from build123d import *

# Parameters (mm, degrees)
SKETCH1_R                    = 3
BOSS_EXTRUDE1_DEPTH          = 10
SKETCH2_R                    = 6
CUT_EXTRUDE1_DEPTH           = 10
SKETCH3_R                    = 52.728139035
CUT_EXTRUDE2_DEPTH           = 10
FILLET1_R                    = 40
SKETCH4_R                    = 2.5
CUT_EXTRUDE3_DEPTH           = 10
CHAMFER1_SIZE                = 2
FILLET2_R                    = 10
LPATTERN3_COUNT              = 5
LPATTERN3_PITCH              = 40
CHAMFER1_OF_LPATTERN3_SIZE   = 2
SKETCH5_R                    = 2.5
CUT_EXTRUDE4_DEPTH           = 10
CHAMFER2_SIZE                = 2
CIRPATTERN2_COUNT            = 45
CHAMFER2_OF_CIRPATTERN2_SIZE = 2
FILLET4_R                    = 82


with BuildPart() as part:
    # Sketch1 → Boss-Extrude1 (new body)
    with BuildSketch(Plane.XY):
        with BuildLine():
            Line((134, -12.3683), (134, -2.7366))
            Line((134, -2.7366), (-66.856482862, -2.7366))
            ThreePointArc((-66.856482862, -2.7366), (-79.305955572, -8.361988007), (-74.83591229, -21.271406043))
            Line((-74.83591229, -21.271406043), (104.205340418, -118.521488224))
            ThreePointArc((104.205340418, -118.521488224), (120.331391511, -85.784656527), (130.366665775, -50.69843496))
            ThreePointArc((130.366665775, -50.69843496), (131.475070851, -44.365109618), (132.383339124, -38))
            ThreePointArc((132.383339124, -38), (133.595433619, -25.209616495), (134, -12.3683))
        make_face()
        with Locations((60, -38)):
            Circle(SKETCH1_R, mode=Mode.SUBTRACT)
        with Locations((-70, -12.3683)):
            Circle(SKETCH1_R, mode=Mode.SUBTRACT)
    extrude(amount=BOSS_EXTRUDE1_DEPTH)

    # Sketch2 → Cut-Extrude1 (cut)
    with BuildSketch(Plane.XY.offset(10)):
        with Locations((60, -38)):
            Circle(SKETCH2_R)
        with Locations((-70, -12.3683)):
            Circle(SKETCH2_R)
    extrude(amount=-CUT_EXTRUDE1_DEPTH, mode=Mode.SUBTRACT)

    # Sketch3 → Cut-Extrude2 (cut)
    with BuildSketch(Plane.XY.offset(10)):
        with Locations((-31.102013179, -89.20992017)):
            Circle(SKETCH3_R)
    extrude(amount=-CUT_EXTRUDE2_DEPTH, mode=Mode.SUBTRACT)

    # Fillet1
    fillet1_edges = [part.edges().sort_by_distance(p)[0] for p in [
        (18.78007916, -72.120932196, 5),
        (-43.920680471, -38.063674805, 5),
    ]]
    fillet(fillet1_edges, radius=FILLET1_R)

    # Sketch4 → Cut-Extrude3 (cut)
    with BuildSketch(Plane.XY.offset(10)):
        with Locations((122, -7.7366)):
            Circle(SKETCH4_R)
    cut_extrude3 = extrude(amount=-CUT_EXTRUDE3_DEPTH, mode=Mode.SUBTRACT)

    # Chamfer1
    chamfer1_edges = [part.edges().sort_by_distance(p)[0] for p in [
        (119.5, -7.7366, 10),
    ]]
    chamfer(chamfer1_edges, length=CHAMFER1_SIZE)

    # Fillet2
    fillet2_edges = [part.edges().sort_by_distance(p)[0] for p in [
        (134, -2.7366, 5),
    ]]
    fillet(fillet2_edges, radius=FILLET2_R)

    # LPattern3: Cut-Extrude3 ×5
    with Locations(*[(-i * LPATTERN3_PITCH, 0, 0) for i in range(1, LPATTERN3_COUNT)]):
        add(cut_extrude3, mode=Mode.SUBTRACT)

    # Chamfer1 of LPattern3
    chamfer1_of_lpattern3_edges = [part.edges().sort_by_distance(p)[0] for p in [
        (79.5, -7.7366, 10),
        (39.5, -7.7366, 10),
        (-0.5, -7.7366, 10),
        (-40.5, -7.7366, 10),
    ]]
    chamfer(chamfer1_of_lpattern3_edges, length=CHAMFER1_OF_LPATTERN3_SIZE)

    # Sketch5 → Cut-Extrude4 (cut)
    with BuildSketch(Plane.XY.offset(10)):
        with Locations((128.565543545, -25.510785173)):
            Circle(SKETCH5_R)
    cut_extrude4 = extrude(amount=-CUT_EXTRUDE4_DEPTH, mode=Mode.SUBTRACT)

    # Chamfer2
    chamfer2_edges = [part.edges().sort_by_distance(p)[0] for p in [
        (126.065543545, -25.510785173, 10),
    ]]
    chamfer(chamfer2_edges, length=CHAMFER2_SIZE)

    # CirPattern2: Cut-Extrude4 ×45 about axis, 41 skipped
    cirpattern2_axis = Axis((-70, -12.3683, 10), (0, 0, 1))
    add([cut_extrude4.rotate(cirpattern2_axis, i * 360 / CIRPATTERN2_COUNT) for i in range(1, CIRPATTERN2_COUNT) if i not in (1, 2, 3, 4, 5, 6, 7, 8, 9, 10, 11, 12, 13, 14, 15, 16, 17, 18, 19, 20, 21, 22, 23, 24, 25, 26, 27, 28, 29, 30, 31, 32, 33, 34, 35, 36, 37, 38, 39, 40, 41)], mode=Mode.SUBTRACT)

    # Chamfer2 of CirPattern2
    chamfer2_of_cirpattern2_edges = [part.edges().sort_by_distance(p)[0] for p in [
        (103.769256405, -104.121598636, 10),
        (114.847737042, -79.044655576, 10),
        (122.328366738, -52.669933097, 10),
    ]]
    chamfer(chamfer2_of_cirpattern2_edges, length=CHAMFER2_OF_CIRPATTERN2_SIZE)

    # Fillet4
    fillet4_edges = [part.edges().sort_by_distance(p)[0] for p in [
        (-66.856482862, -2.7366, 5),
    ]]
    fillet(fillet4_edges, radius=FILLET4_R)


solid = part.part
Geometry check sheet. Reference: the model listing, model coordinates, mm. Give positions to 0.01 mm unless a question says otherwise; leave off trailing zeros. Order: outer loops, then holes, each group sorted by start corner. A loop starts at its lowest first (then second) coordinate and runs counter-clockwise, first axis right, second up. Notation, with made-up numbers: M 74.25,-29 L 90.25,-29 A10 cw 90.25,-11 Z; hole C 14.25,61 d5. An arc over 180 degrees is marked long. Use a Markdown table: item, result.
Item 1: Draft check along X on faces 1 (the cylindrical face through (0.02, -9.26, 4.06)), 2 (the flat face through (33, -2.737, 5)), 3 (the flat face through (66.76, -98.18, 4.93)). Enter one of: +X half, -X half, draft (parallel to the pull), parting line (faces both ways), or undercut.
Answers follow:
| item | result |
|---|---|
| face 1 | undercut |
| face 2 | draft |
| face 3 | -X half |
Item 2: Depth check by flat-ended pin: P1, Ø3, axis at x = -38, y = -7.74, coming from the -Z side; P2, Ø2, axis at x = 65, y = -39.5, coming from the -Z side; P3, Ø1, axis at y = -64, z = 7, coming from the +X side; P4, Ø3, axis at y = -55, z = 3.5, coming from the +X side. Enter the tip coordinate at first touch or a pass-through.
Answers follow:
| item | result |
|---|---|
| P1 | passes through |
| P2 | stops at z = 0 |
| P3 | stops at x = 127.49 |
| P4 | stops at x = 129.81 |
Item 3: Section check A-A (x = 42). Record the cut outline in (y, z).
Answers follow:
| item | result |
|---|---|
| outline | M -84.73,0 L -10.24,0 L -10.24,8 L -12.24,10 L -84.73,10 Z; M -5.24,0 L -2.74,0 L -2.74,10 L -3.24,10 L -5.24,8 Z |
Item 4: Material ranges on line 1 along Y through (x, z) = (107, 9.5); line 2 along Y through (x, z) = (2, 6.25); line 3 along X through (y, z) = (-17.5, 2.5), recorded low to high.
Answers follow:
| item | result |
|---|---|
| line 1 | y = -113.79 to -109.02, -101.25 to -2.74 |
| line 2 | y = -48.17 to -10.24, -5.24 to -2.74 |
| line 3 | x = -78.74 to -73.11, -66.89 to 133.94 |
Item 5: Section check B-B (x = 2). Record the cut outline in (y, z).
Answers follow:
| item | result |
|---|---|
| outline | M -48.17,0 L -10.24,0 L -10.24,8 L -12.24,10 L -48.17,10 Z; M -5.24,0 L -2.74,0 L -2.74,10 L -3.24,10 L -5.24,8 Z |
Item 6: Section check C-C (x = -45). Record the cut outline in (y, z), and give its area (3 significant figures).
Answers follow:
| item | result |
|---|---|
| outline | M -35.7,0 L -2.74,0 L -2.74,10 L -35.7,10 Z |
| area | 330 mm2 |
